from build123d import *

# Parameters (mm, degrees)
BOSS_EXTRUDE1_DEPTH                      = 30
SKETCH2_W                                = 30
SKETCH2_H                                = 30
BOSS_EXTRUDE2_DEPTH                      = 10
SKETCH3_R                                = 65
BOSS_EXTRUDE3_DEPTH                      = 3
SKETCH4_R                                = 30
BOSS_EXTRUDE4_DEPTH                      = 10
CBORE_FOR_M6_PAN_HEAD_SCREW1_D           = 6.6
CBORE_FOR_M6_PAN_HEAD_SCREW1_DEPTH       = 50.5
CBORE_FOR_M6_PAN_HEAD_SCREW1_CBORE_D     = 13
CBORE_FOR_M6_PAN_HEAD_SCREW1_CBORE_DEPTH = 4.6
CBORE_FOR_M6_PAN_HEAD_SCREW1_TIP         = 1.982840043


with BuildPart() as part:
    # Sketch1 → Boss-Extrude1 (new body)
    with BuildSketch(Plane.XY):
        with BuildLine():
            Line((12.115384439, 172.009473486), (-71.801857106, 194.602576649))
            ThreePointArc((-71.801857106, 194.602576649), (-160, 127.009473486), (-71.801857106, 59.416370323))
            Line((-71.801857106, 59.416370323), (12.115384439, 82.009473486))
            ThreePointArc((12.115384439, 82.009473486), (46.602387708, 127.009473486), (12.115384439, 172.009473486))
        make_face()
    extrude(amount=BOSS_EXTRUDE1_DEPTH)

    # Sketch2 → Boss-Extrude2 (add)
    with BuildSketch(Plane(origin=(0, 0, 0), x_dir=(-1, 0, 0), z_dir=(0, 0, -1))):
        with Locations((90, 127.009473486)):
            Rectangle(SKETCH2_W, SKETCH2_H)
    extrude(amount=BOSS_EXTRUDE2_DEPTH)

    # Sketch3 → Boss-Extrude3 (add)
    with BuildSketch(Plane.XY.offset(30)):
        with Locations((-90, 127.009473486)):
            Circle(SKETCH3_R)
    extrude(amount=BOSS_EXTRUDE3_DEPTH)

    # Sketch4 → Boss-Extrude4 (add)
    with BuildSketch(Plane.XY.offset(33)):
        with Locations((-90, 127.009473486)):
            Circle(SKETCH4_R)
    extrude(amount=BOSS_EXTRUDE4_DEPTH)

    # CBORE for M6 Pan Head Screw1
    with Locations(Plane(origin=(12.115384439, 157.009473486, 30), x_dir=(1, 0, 0), z_dir=(0, 0, 1))):
        with Locations((0, 0), (0, -60)):
            CounterBoreHole(CBORE_FOR_M6_PAN_HEAD_SCREW1_D / 2, CBORE_FOR_M6_PAN_HEAD_SCREW1_CBORE_D / 2, CBORE_FOR_M6_PAN_HEAD_SCREW1_CBORE_DEPTH, depth=CBORE_FOR_M6_PAN_HEAD_SCREW1_DEPTH)
            with Locations((0, 0, -(CBORE_FOR_M6_PAN_HEAD_SCREW1_DEPTH + CBORE_FOR_M6_PAN_HEAD_SCREW1_TIP / 2))):  # 118° drill point
                Cone(0, CBORE_FOR_M6_PAN_HEAD_SCREW1_D / 2, CBORE_FOR_M6_PAN_HEAD_SCREW1_TIP, mode=Mode.SUBTRACT)


solid = part.part
For this review, take the finished solid that the model builds, in its own axes (mm). A direction names the side the tool comes from. Give positions to 0.01 mm unless a question says otherwise; leave off trailing zeros. Loops run counter-clockwise (first coordinate to the right, second up) from the corner with the lowest first, then second, coordinate; pieces in that order, holes last. Notation, with made-up numbers: M -4,-38.5 L 28,-38.5 A37 cw 28,-1.5 Z; hole C 40,11 d2. An arc over 180 degrees is marked long. Answer as a JSON object with one key per item and string values. Group by question number.
Q1. For probe 1 along Z at (x, y) = (-100, 181); probe 2 along X at (y, z) = (162, 27.5); probe 3 along Z at (x, y) = (7, 94), list the stretches that pass through material, from the lowest coordinate up. Write a range as [from, to].
Q2. Insertion check: P1, Ø15, axis at x = 12.12, y = 157.01, coming from the +Z side; P2, Ø3, axis at x = -92.5, z = -6, coming from the +Y side; P3, Ø6, axis at x = 9.5, y = 89, coming from the -Z side. Each pin has a flat end and moves straight along its axis. Give the tip position at first contact, or say it passes through.
Q3. Add section B-B on x = -90. Give the boundary of the cut face in (y, z), and give its area (3 significant figures).
Q4. Mouldability with a two-part tool opening along Y and no side actions: class faces 1 (the cylindrical face through (-98.462, 191.456, 31.479)), 2 (the cylindrical face through (9.067, 155.746, 12.522)), 3 (the flat face through (-90, 142.009, -5)) as +Y half, -Y half, draft (parallel to the pull), parting line (faces both ways), or undercut.
Q5. Add section C-C on y = 146. Give the boundary of the cut face in (x, z).
Q6. Tool access review of faces 4 (the flat face through (-76, 99, 33)), 5 (the flat face through (-75, 127, -5)), 6 (the flat face through (-90, 112.009, -5)), 7 (the flat face through (-105, 127, -5)): name each direction out of +Z, -Z, +X, -X, +Y, -Y from which nothing blocks a thin tool from reaching the whole face with its end or side.
Q7. Add section A-A on z = 11. Give the boundary of the cut face in (x, y).
Q8. Add section D-D on y = 178. Give the boundary of the cut face in (x, z).
Checked values:
{
 "1": {"probe 1": "[0, 33]", "probe 2": "[-150.63, 7.95], [16.28, 30.78]", "probe 3": "[0, 25.4]"},
 "2": {"P1": "z = 30", "P2": "y = 142.01", "P3": "z = 0"},
 "3": {"outline": "M 57.01,0 L 112.01,0 L 112.01,-10 L 142.01,-10 L 142.01,0 L 197.01,0 L 197.01,30 L 192.01,30 L 192.01,33 L 157.01,33 L 157.01,43 L 97.01,43 L 97.01,33 L 62.01,33 L 62.01,30 L 57.01,30 Z", "area": "5,490 mm²"},
 "4": {"face 1": "parting line", "face 2": "undercut", "face 3": "+Y half"},
 "5": {"outline": "M -157.37,0 L 42.56,0 L 42.56,30 L -27.84,30 L -27.84,33 L -66.78,33 L -66.78,43 L -113.22,43 L -113.22,33 L -152.16,33 L -152.16,30 L -157.37,30 Z"},
 "6": {"face 4": "+Z", "face 5": "-Z, +X, +Y, -Y", "face 6": "-Z, +X, -X, -Y", "face 7": "-Z, -X, +Y, -Y"},
 "7": {"outline": "M -71.8,59.42 L 12.12,82.01 A46.6 ccw 12.12,172.01 L -71.8,194.6 A70 ccw long Z; hole C 12.12,97.01 d6.6; hole C 12.12,157.01 d6.6"},
 "8": {"outline": "M -137.96,0 L -10.14,0 L -10.14,30 L -49.69,30 L -49.69,33 L -130.31,33 L -130.31,30 L -137.96,30 Z"}
}
